Input: dimensioned drawing with shaded views. Units: mm. Origin: part minimum x, y, z. Give positions to 0.01 mm unless a question says otherwise; leave off trailing zeros. Write each loop counter-clockwise with the first axis right and the second up, starting at its lowest first coordinate (ties: lowest second). Pieces come first, ordered by that corner, then holes.
Q1. Section C-C (x = 0.6). Return the cut outline in (y, z).
Q2. Line query: line 1 (X direction, y = 3.35, z = 22.5); line 2 (Y direction, x = 1.2, z = 16); line 3 (X direction, y = 1.85, z = 22.5). Output: solid intervals per line, ascending.
Q3. Section A-A (y = 3.2). Return the cut outline in (x, z), plus the area to 3 significant figures.
Q4. Pin query (flat end, axial travel): pin 1 Ø1.5 at (y, z) = (0.5, 26.5) entering from +X. Return the tip coordinate at first contact, or that it passes through.
Q5. Section B-B (z = 37). Return the cut outline in (x, y).
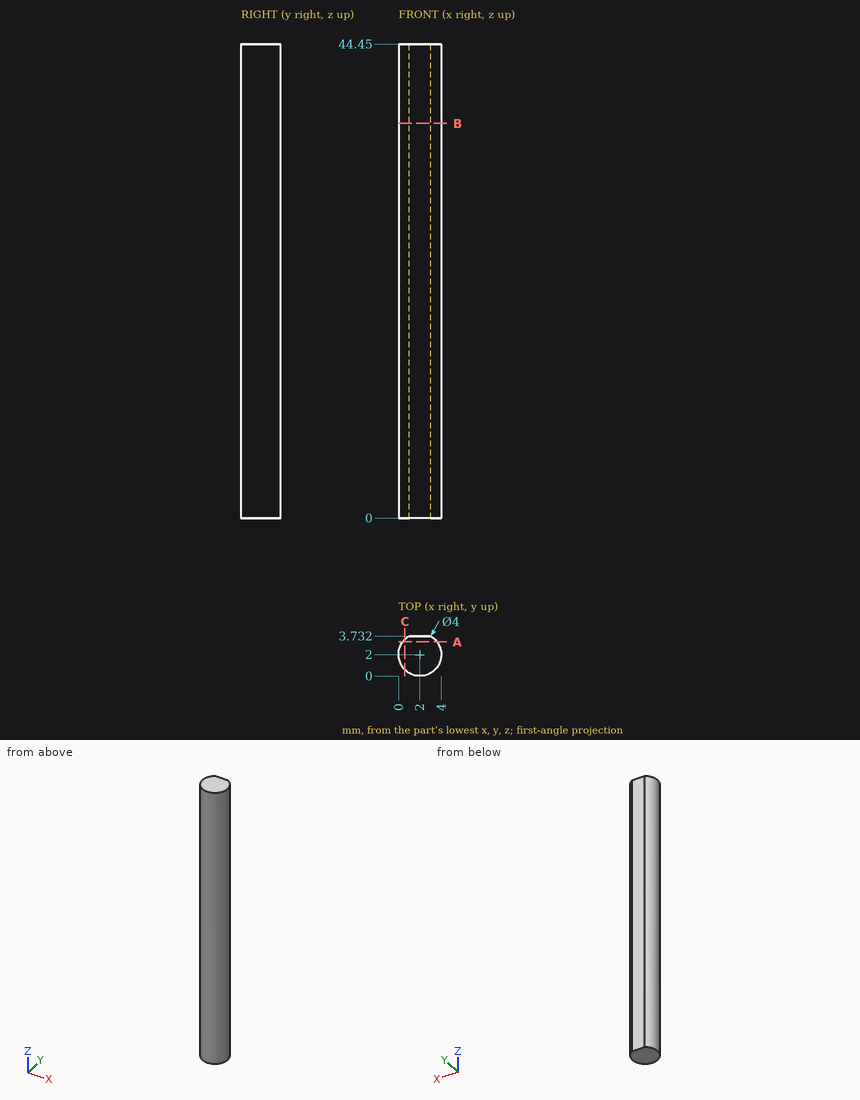
Computed:
1. outline: (0.57, 0) - (3.43, 0) - (3.43, 44.45) - (0.57, 44.45) - close
2. line 1: x = 0.52 to 3.48
2. line 2: y = 0.17 to 3.73
2. line 3: x = 0.01 to 3.99
3. outline: (0.4, 0) - (3.6, 0) - (3.6, 44.45) - (0.4, 44.45) - close
3. area: 142 mm2
4. pin 1: stops at x = 3.85
5. outline: (1, 3.73) arc R2 ccw (long way) to (3, 3.73) - close
